Design review of the part shown in the three views and the two pictorial views. Dimensions are in mm from the part's minimum x, y and z. A direction names the side the tool comes from. Give positions to 0.01 mm unless a question says otherwise; leave off trailing zeros. Order: outer loops, then holes, each group sorted by start corner. A loop starts at its lowest first (then second) coordinate and runs counter-clockwise, first axis right, second up.
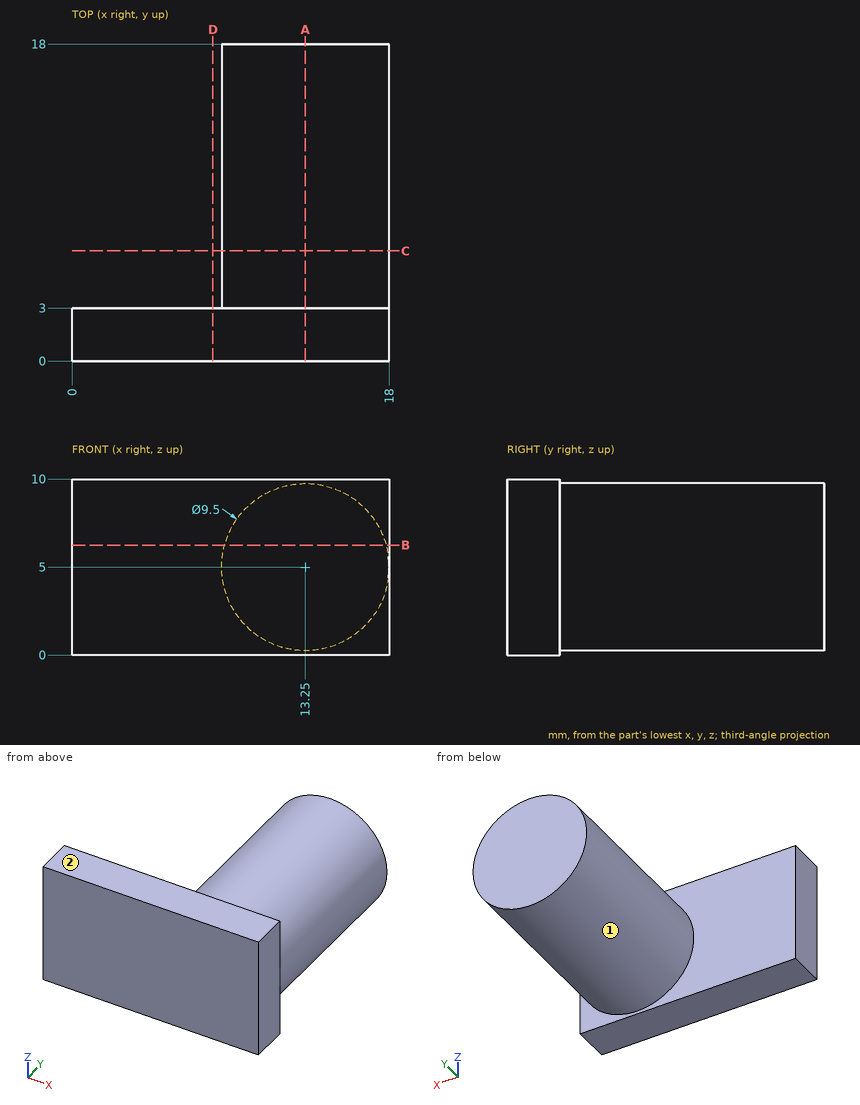
1) Tool access review of the marked faces 1 and 2: name each direction out of +Z, -Z, +X, -X, +Y, -Y from which nothing blocks a thin tool from reaching the whole face with its end or side.
Answer sheet:
face 1: +Y
face 2: +Z, +X, -X, +Y, -Y
2) Clearance check with flat-ended pins moving along their axes: pin 1 (5 mm diameter, centred on x = 2, z = 2, fed in from +Y); pin 2 (1.5 mm diameter, centred on y = 5, z = 1.5, fed in from -X). State where each tip first meets the part, or that it passes through.
Answer sheet:
pin 1: stops at y = 3
pin 2: stops at x = 9.38
3) We need section D-D on x = 8. Give the boundary of the cut face in (y, z), then the cut area to 3 significant figures.
Answer sheet:
outline: (0, 0) - (3, 0) - (3, 10) - (0, 10) - close
area: 30.0 mm2
4) We need section B-B on z = 6.25. Give the boundary of the cut face in (x, y).
Answer sheet:
outline: (0, 0) - (18, 0) - (18, 3) - (17.83, 3) - (17.83, 18) - (8.67, 18) - (8.67, 3) - (0, 3) - close
5) We need section C-C on y = 6.25. Give the boundary of the cut face in (x, z), then the cut area to 3 significant figures.
Answer sheet:
outline: circle Ø9.5 at (13.25, 5)
area: 70.9 mm2
6) To check wall thickness, follow line 1 (Y direction, x = 16.75, z = 9.5); line 2 (Z direction, x = 10.75, y = 15.75); line 3 (Z direction, x = 16.5, y = 14.5). State the ranges of each line that lie inside material, in increasing order.
Answer sheet:
line 1: y = 0 to 3
line 2: z = 0.96 to 9.04
line 3: z = 1.54 to 8.46
7) We need section A-A on x = 13.25. Give the boundary of the cut face in (y, z).
Answer sheet:
outline: (0, 0) - (3, 0) - (3, 0.25) - (18, 0.25) - (18, 9.75) - (3, 9.75) - (3, 10) - (0, 10) - close
